Read the model definition and answer for the solid it produces. Units are mm, in the model's axes. Round coordinates to 2 decimals unless told otherwise and drop trailing zeros. Order: outer loops, then holes, each group sorted by start corner. A loop starts at its lowest first (then second) coordinate and runs counter-clockwise, first axis right, second up. Notation, with made-up numbers: (47, -10) - (51, -10) arc R34 ccw to (51, 22) - close; hole circle Ø3 at (44.5, 47). An arc over 180 degrees is marked (long way). One line per question, with ' | ' between items. Start each with the question number.
1) Straight lines are drawn through the part: line 1 (X direction, y = 35, z = 2.4); line 2 (Y direction, x = 32.5, z = 1.65); line 3 (Y direction, x = -2, z = 4.45). For each, find the intervals that lie inside material, in ascending order. Write a range as from..to.
2) The part is cut by section A-A, the plane z = 1.85. Give the vertices of the cut face in (x, y), plus the area to 3 significant figures.
3) The part is cut by section B-B, the plane x = 22. Give the vertices of the cut face in (y, z).
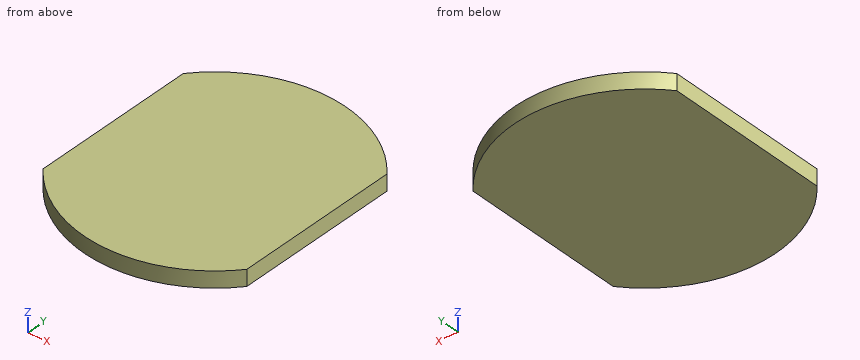
from build123d import *

# Parameters (mm, degrees)
SKETCH_1_R     = 45
PAD_1_DEPTH    = 5.5
SKETCH_2_W     = 15
SKETCH_2_H     = 100
POCKET_2_DEPTH = 5.501
SKETCH_3_W     = 15
SKETCH_3_H     = 100
POCKET_3_DEPTH = 5.501


with BuildPart() as part:
    # Sketch_1 → Pad_1 (new body)
    with BuildSketch(Plane.XY):
        Circle(SKETCH_1_R)
    extrude(amount=PAD_1_DEPTH)

    # Sketch_2 (on Face3 of Pad_1) → Pocket_2 (cut, through all)
    with BuildSketch(Plane.XY.offset(5.5)):
        with Locations((-42.5, 0)):
            Rectangle(SKETCH_2_W, SKETCH_2_H)
    extrude(amount=-POCKET_2_DEPTH, mode=Mode.SUBTRACT)

    # Sketch_3 (on Face3 of Pocket_2) → Pocket_3 (cut, through all)
    with BuildSketch(Plane.XY.offset(5.5)):
        with Locations((42.5, 0)):
            Rectangle(SKETCH_3_W, SKETCH_3_H)
    extrude(amount=-POCKET_3_DEPTH, mode=Mode.SUBTRACT)


solid = part.part
Values:
1) line 1: x = -28.28..28.28 | line 2: y = -31.12..31.12 | line 3: y = -44.96..44.96
2) outline: (-35, -28.28) arc R45 ccw to (35, -28.28) - (35, 28.28) arc R45 ccw to (-35, 28.28) - close | area: 5,590 mm^2
3) outline: (-39.26, 0) - (39.26, 0) - (39.26, 5.5) - (-39.26, 5.5) - close
